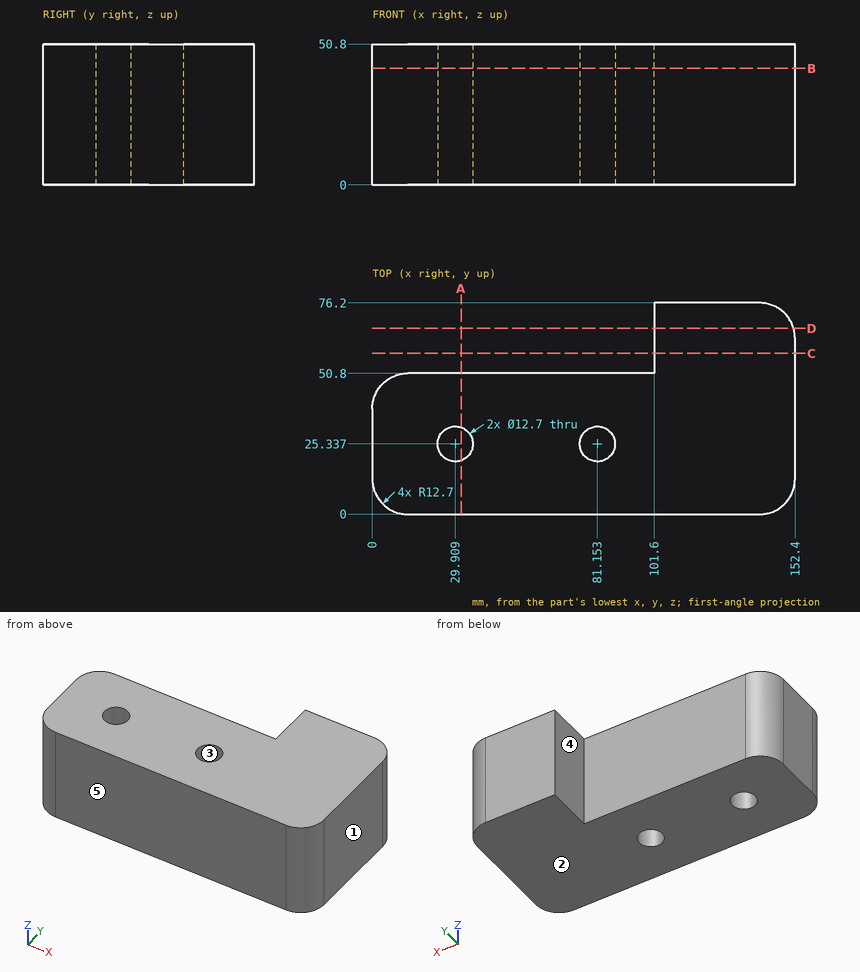
The figure shows three views and two pictorial views of one solid part (mm, origin at its lowest corner). Answer the questions. A direction names the side the tool comes from. Round coordinates to 2 decimals unless told otherwise and drop trailing zeros. Write each loop counter-clockwise with the first axis right and the second up, starting at its lowest first coordinate (ties: lowest second). Pieces come first, ordered by that corner, then holes. Notation, with made-up numbers: (-10.75, 10.5) - (6.25, 10.5) arc R30 cw to (6.25, 45.5) - close; hole circle Ø3 at (-6.75, 20). An arc over 180 degrees is marked (long way). Use one line per item in the form item = value. Start each with the question number.
Item 1: A flat-ended cylindrical pin translates along its axis: pin 1 Ø2 at (y, z) = (57.5, 27) entering from -X. Find the tip coordinate at first contact, or state that the pin passes through.
Item 2: Find the intervals of material crossed by line 1 (Y direction, x = 30, z = 34.5) (1 decimal); line 2 (X direction, y = 28, z = 21) (1 decimal); line 3 (X direction, y = 24, z = 30) (1 decimal), in increasing order. Write a range as [from, to].
Item 3: A tool of negligible diameter and unlimited length cuts with its end or side. For the marked faces 4 and 5, from which of +Z, -Z, +X, -X, +Y, -Y can it reach the whole face along a straight path? Write none if from no direction.
Item 4: A cutting plane is placed at D-D (y = 67). Write down the section's boundary in (x, z).
Item 5: Determine the mould class of the marked faces 1, 2 and 3 for opening direction X: +X half, -X half, draft (parallel to the pull), parting line (faces both ways), or undercut.
Item 6: A cutting plane is placed at C-C (y = 58). Write down the section's boundary in (x, z), plus the area to 3 significant figures.
Item 7: A cutting plane is placed at A-A (x = 32). Write down the section's boundary in (y, z).
Item 8: A cutting plane is placed at B-B (z = 42). Write down the section's boundary in (x, y), plus the area to 3 significant figures.
The answers:
q1.pin_1 = 101.6
q2.line_1 = [0, 19], [31.7, 50.8]
q2.line_2 = [0, 24.1], [35.7, 75.4], [86.9, 152.4]
q2.line_3 = [0, 23.7], [36.1, 74.9], [87.4, 152.4]
q3.face_4 = +Z, -Z, -X, +Y
q3.face_5 = +Z, -Z, +X, -X, -Y
q4.outline = (101.6, 0) - (151.91, 0) - (151.91, 50.8) - (101.6, 50.8) - close
q5.face_1 = +X half
q5.face_2 = draft
q5.face_3 = undercut
q6.outline = (101.6, 0) - (152.4, 0) - (152.4, 50.8) - (101.6, 50.8) - close
q6.area = 2,580 mm^2
q7.outline = (0, 0) - (19.34, 0) - (19.34, 50.8) - (0, 50.8) - close; (31.33, 0) - (50.8, 0) - (50.8, 50.8) - (31.33, 50.8) - close
q8.outline = (0, 12.7) arc R12.7 ccw to (12.7, 0) - (139.7, 0) arc R12.7 ccw to (152.4, 12.7) - (152.4, 63.5) arc R12.7 ccw to (139.7, 76.2) - (101.6, 76.2) - (101.6, 50.8) - (12.7, 50.8) arc R12.7 ccw to (0, 38.1) - close; hole circle Ø12.7 at (29.91, 25.34); hole circle Ø12.7 at (81.15, 25.34)
q8.area = 8,640 mm^2
